Build history of the part. All positions in model axes, mm. A direction names the side the tool comes from. Round coordinates to 2 decimals unless told otherwise and drop trailing zeros. Write each loop counter-clockwise with the first axis right and the second up, starting at its lowest first coordinate (ties: lowest second). Pieces come first, ordered by that corner, then holes.
from build123d import *

# Parameters (mm, degrees)
BOSS_EXTRUDE1_DEPTH = 1.8
SKETCH2_W           = 12
SKETCH2_H           = 3.5
CUT_EXTRUDE1_DEPTH  = 0.6
SKETCH3_R           = 3
BOSS_EXTRUDE2_DEPTH = 4.2
SKETCH4_R           = 0.8
CUT_EXTRUDE2_DEPTH  = 15.920922753


with BuildPart() as part:
    # Sketch1 → Boss-Extrude1 (new body)
    with BuildSketch(Plane(origin=(0, 0, 0), x_dir=(1, 0, 0), z_dir=(0, 1, 0))):
        with BuildLine():
            Line((-3.465517241, 4.74137931), (8.534482759, 4.74137931))
            Line((8.534482759, 4.74137931), (8.534482759, -5.25862069))
            ThreePointArc((8.534482759, -5.25862069), (2.534482759, -11.25862069), (-3.465517241, -5.25862069))
            Line((-3.465517241, -5.25862069), (-3.465517241, 4.74137931))
        make_face()
    extrude(amount=BOSS_EXTRUDE1_DEPTH)

    # Sketch2 → Cut-Extrude1 (cut)
    with BuildSketch(Plane(origin=(0, 1.8, 0), x_dir=(1, 0, 0), z_dir=(0, 1, 0))):
        with Locations((2.534482759, 2.99137931)):
            Rectangle(SKETCH2_W, SKETCH2_H)
    extrude(amount=-CUT_EXTRUDE1_DEPTH, mode=Mode.SUBTRACT)

    # Sketch3 → Boss-Extrude2 (add)
    with BuildSketch(Plane(origin=(0, 1.8, 0), x_dir=(1, 0, 0), z_dir=(0, 1, 0))):
        with Locations(Location((2.534482759, -5.25862069, 0), (0, 0, 270))):
            Circle(SKETCH3_R)
    extrude(amount=BOSS_EXTRUDE2_DEPTH)

    # Sketch4 → Cut-Extrude2 (cut, through all)
    with BuildSketch(Plane(origin=(0, 1.2, 0), x_dir=(1, 0, 0), z_dir=(0, 1, 0))):
        with Locations(Location((5.534482759, 2.99137931, 0), (0, 0, 270))):
            Circle(SKETCH4_R)
        with Locations(Location((-0.465517241, 2.99137931, 0), (0, 0, 90))):
            Circle(SKETCH4_R)
    extrude(amount=-CUT_EXTRUDE2_DEPTH, mode=Mode.SUBTRACT)


solid = part.part
1) Mould opens along X. For faces 1 (the cylindrical face through (-0.501, 0.608, -2.192)), 2 (the flat face through (8.534, 1, 0)), 3 (the flat face through (2, 1, -4.741)) say: released by +X, released by -X, zero draft, split by the parting line, or undercut.
Results:
face 1: undercut
face 2: released by +X
face 3: zero draft
2) Slice it at A-A (y = 0.75). Write the cut outline in (x, z).
Results:
outline: (-3.47, -4.74) - (8.53, -4.74) - (8.53, 5.26) arc R6 ccw to (-3.47, 5.26) - close; hole circle Ø1.6 at (-0.47, -2.99); hole circle Ø1.6 at (5.53, -2.99)
3) Slice it at C-C (z = -1.5). Write the cut outline in (x, y).
Results:
outline: (-3.47, 0) - (8.53, 0) - (8.53, 1.2) - (-3.47, 1.2) - close
4) Which spindle directions (+Z, -Z, +X, -X, +Y, -Y) get a long thin tool onto all of the face, cutting with end or side? Do faces 4 (the cylindrical face through (1.39, 3.87, 8.03)), 5 (the cylindrical face through (2.666, 0.887, 11.257)), 6 (the flat face through (2, 1.2, -3)). Say none if no direction does.
Results:
face 4: +Y
face 5: +Z, +Y, -Y
face 6: -Z, +X, -X, +Y
5) Slice it at D-D (x = 3.5). Write the cut outline in (y, z), plus the area to 3 significant figures.
Results:
outline: (0, -4.74) - (1.2, -4.74) - (1.2, -1.24) - (1.8, -1.24) - (1.8, 2.42) - (6, 2.42) - (6, 8.1) - (1.8, 8.1) - (1.8, 11.18) - (0, 11.18) - close
area: 50.4 mm2
6) Pin check, flat tips, straight feed: pin 1 Ø2 at (x, y) = (4, 4) entering from +Z; pin 2 Ø3 at (x, z) = (2, -3.5) entering from +Y; pin 3 Ø0.5 at (x, y) = (5, 1.5) entering from -Z. Stop position of each tip, or through.
Results:
pin 1: stops at z = 8.22
pin 2: stops at y = 1.2
pin 3: stops at z = -1.24
7) Wall check: L1, parallel to Y at x = 2.5, z = 9.75; L2, parallel to Y at x = 5.5, z = -1.75; L3, parallel to Z at x = 4.75, y = 5.5. Give the ranges that are in metal, low to high.
Results:
L1: y = 0 to 1.8
L2: y = 0 to 1.2
L3: z = 3.24 to 7.28
8) Slice it at B-B (x = -1). Write the cut outline in (y, z), plus the area to 3 significant figures.
Results:
outline: (0, -4.74) - (1.2, -4.74) - (1.2, -3.59) - (0, -3.59) - close; (0, -2.4) - (1.2, -2.4) - (1.2, -1.24) - (1.8, -1.24) - (1.8, 10.11) - (0, 10.11) - close
area: 23.2 mm2
